from build123d import *

# Parameters (mm, degrees)
BOSS_EXTRUDE1_DEPTH                                = 4
CUT_EXTRUDE1_DEPTH                                 = 3
CUT_EXTRUDE2_DEPTH                                 = 58.329679868
F_3_2_3_2_DIAMETER_HOLE1_D                         = 3.2
F_3_2_3_2_DIAMETER_HOLE1_DEPTH                     = 6
CBORE_FOR_M3_5_HEX_HEAD_MACHINE_SCREW1_D           = 4
CBORE_FOR_M3_5_HEX_HEAD_MACHINE_SCREW1_CBORE_D     = 8
CBORE_FOR_M3_5_HEX_HEAD_MACHINE_SCREW1_CBORE_DEPTH = 4.5
CHAMFER1_SIZE                                      = 1.55
CHAMFER2_SIZE                                      = 0.799999982
CHAMFER2_SIZE2                                     = 0.800000027
CHAMFER3_SIZE                                      = 0.799999997
CHAMFER3_SIZE2                                     = 0.800000017
FILLET1_R                                          = 3
FILLET2_R                                          = 4.1
FILLET3_R                                          = 5
FILLET4_R                                          = 5.100000015


with BuildPart() as part:
    # Sketch1 → Boss-Extrude1 (new body)
    with BuildSketch(Plane(origin=(0, 4, 0), x_dir=(1, 0, 0), z_dir=(0, 1, 0))):
        with BuildLine():
            Line((19.999999925, -16.999999746), (19.999999925, 25.309401343))
            Line((19.999999925, 25.309401343), (29.980761952, 31.071796677))
            ThreePointArc((29.980761952, 31.071796677), (32.90896539, 41.999999919), (21.980762114, 44.92820323))
            Line((21.980762114, 44.92820323), (12.345871038, 39.365496274))
            ThreePointArc((12.345871038, 39.365496274), (0, 43.5), (-12.345871038, 39.365496274))
            Line((-12.345871038, 39.365496274), (-21.980762114, 44.92820323))
            ThreePointArc((-21.980762114, 44.92820323), (-32.908965409, 41.999999887), (-29.980761888, 31.071796639))
            Line((-29.980761888, 31.071796639), (-19.999999289, 25.3094011))
            Line((-19.999999289, 25.3094011), (-19.999999289, -16.999999746))
            Line((-19.999999289, -16.999999746), (19.999999925, -16.999999746))
        make_face()
    extrude(amount=-BOSS_EXTRUDE1_DEPTH)

    # Sketch2 → Cut-Extrude1 (cut)
    with BuildSketch(Plane(origin=(0, 4, 0), x_dir=(-1, 0, 0), z_dir=(0, 1, 0))):
        with BuildLine():
            Line((-4.968651732, -32.250000015), (4.968651732, -32.250000015))
            ThreePointArc((4.968651732, -32.250000015), (10.500000015, -23), (4.968651732, -13.749999985))
            Line((4.968651732, -13.749999985), (-4.968651732, -13.749999985))
            ThreePointArc((-4.968651732, -13.749999985), (-10.500000015, -23), (-4.968651732, -32.250000015))
        make_face()
    extrude(amount=-CUT_EXTRUDE1_DEPTH, mode=Mode.SUBTRACT)

    # Sketch3 → Cut-Extrude2 (cut, through all)
    with BuildSketch(Plane.XZ):
        with BuildLine():
            Line((4.71036092, -14.75), (-4.71036092, -14.75))
            ThreePointArc((-4.71036092, -14.75), (-9.5, -23), (-4.71036092, -31.25))
            Line((-4.71036092, -31.25), (4.71036092, -31.25))
            ThreePointArc((4.71036092, -31.25), (9.5, -23), (4.71036092, -14.75))
        make_face()
    extrude(amount=-CUT_EXTRUDE2_DEPTH, mode=Mode.SUBTRACT)

    # Sketch4 → Revolve1 (revolve)
    with BuildSketch(Plane(origin=(0, 0, -38), x_dir=(-1, 0, 0), z_dir=(0, 0, -1)), mode=Mode.PRIVATE) as revolve1_sk:
        Polygon((18.980762114, 4), (25.980762114, 4), (25.980762114, 6), (19.980762114, 6), (18.980762114, 5), align=None)
    revolve(revolve1_sk.sketch.rotate(Axis((-25.980762114, 4, -38), (0, 1, 0)), 270), axis=Axis((-25.980762114, 4, -38), (0, 1, 0)))

    # Sketch5 → Revolve2 (revolve)
    with BuildSketch(Plane(origin=(0, 0, 7), x_dir=(-1, 0, 0), z_dir=(0, 0, -1)), mode=Mode.PRIVATE) as revolve2_sk:
        Polygon((-7, 4), (0, 4), (0, 6), (-6, 6), (-7, 5), align=None)
    revolve(revolve2_sk.sketch.rotate(Axis((0, 4, 7), (0, 1, 0)), 180), axis=Axis((0, 4, 7), (0, 1, 0)))

    # Sketch6 → Revolve3 (revolve)
    with BuildSketch(Plane(origin=(0, 0, -38), x_dir=(-1, 0, 0), z_dir=(0, 0, -1)), mode=Mode.PRIVATE) as revolve3_sk:
        Polygon((-32.980762114, 4), (-25.980762114, 4), (-25.980762114, 6), (-31.980762114, 6), (-32.980762114, 5), align=None)
    revolve(revolve3_sk.sketch.rotate(Axis((25.980762114, 4, -38), (0, 1, 0)), 270), axis=Axis((25.980762114, 4, -38), (0, 1, 0)))

    # Ø3.2 (3.2) Diameter Hole1
    with Locations(Plane(origin=(0, 0, 0), x_dir=(-1, 0, 0), z_dir=(0, -1, 0))):
        with Locations((15.000000337, 33.000000191), (-14.999999663, 10.500000191), (15.000000337, -11.999999809), (-14.999999663, -11.999999809), (15.000000337, 10.500000191), (-14.999999663, 33.000000191)):
            Hole(F_3_2_3_2_DIAMETER_HOLE1_D / 2, depth=F_3_2_3_2_DIAMETER_HOLE1_DEPTH)

    # CBORE for M3.5 Hex Head Machine Screw1 (through all)
    with Locations(Plane(origin=(0, 0, 0), x_dir=(-1, 0, 0), z_dir=(0, -1, 0))):
        with Locations((0, -7), (-25.980762114, 38), (25.980762114, 38)):
            CounterBoreHole(CBORE_FOR_M3_5_HEX_HEAD_MACHINE_SCREW1_D / 2, CBORE_FOR_M3_5_HEX_HEAD_MACHINE_SCREW1_CBORE_D / 2, CBORE_FOR_M3_5_HEX_HEAD_MACHINE_SCREW1_CBORE_DEPTH)

    # Chamfer1
    chamfer1_edges = [part.edges().sort_by_distance(p)[0] for p in [
        (13.399999663, 0, -10.500000191),
        (-16.600000337, 0, -33.000000191),
        (13.399999663, 0, -33.000000191),
        (-16.600000337, 0, -10.500000191),
        (13.399999663, 0, 11.999999809),
        (-16.600000337, 0, 11.999999809),
    ]]
    chamfer(chamfer1_edges, length=CHAMFER1_SIZE)

    # Chamfer2
    chamfer2_edges = [part.edges().sort_by_distance(p)[0] for p in [
        (-19.999999289, 2, 16.999999746),
    ]]
    chamfer2_side = [part.faces().sort_by_distance(p)[0] for p in [
        (3.18e-07, 2, 16.999999746),
    ]]
    chamfer(chamfer2_edges, length=CHAMFER2_SIZE, length2=CHAMFER2_SIZE2, reference=chamfer2_side[0])

    # Chamfer3
    chamfer3_edges = [part.edges().sort_by_distance(p)[0] for p in [
        (19.999999925, 2, 16.999999746),
    ]]
    chamfer3_side = [part.faces().sort_by_distance(p)[0] for p in [
        (0.400000309, 2, 16.999999746),
    ]]
    chamfer(chamfer3_edges, length=CHAMFER3_SIZE, length2=CHAMFER3_SIZE2, reference=chamfer3_side[0])

    # Fillet1
    fillet1_edges = [part.edges().sort_by_distance(p)[0] for p in [
        (-12.345871038, 2, -39.365496274),
        (12.345871038, 2, -39.365496274),
    ]]
    fillet(fillet1_edges, radius=FILLET1_R)

    # Fillet2
    fillet2_edges = [part.edges().sort_by_distance(p)[0] for p in [
        (4.71036092, 0.5, -14.75),
        (4.71036092, 0.5, -31.25),
        (-4.71036092, 0.5, -31.25),
        (-4.71036092, 0.5, -14.75),
    ]]
    fillet(fillet2_edges, radius=FILLET2_R)

    # Fillet3
    fillet3_edges = [part.edges().sort_by_distance(p)[0] for p in [
        (-19.999999289, 2, -25.3094011),
        (19.999999925, 2, -25.309401343),
    ]]
    fillet(fillet3_edges, radius=FILLET3_R)

    # Fillet4
    fillet4_edges = [part.edges().sort_by_distance(p)[0] for p in [
        (4.968651732, 2.5, -32.250000015),
        (4.968651732, 2.5, -13.749999985),
        (-4.968651732, 2.5, -13.749999985),
        (-4.968651732, 2.5, -32.250000015),
    ]]
    fillet(fillet4_edges, radius=FILLET4_R)


solid = part.part
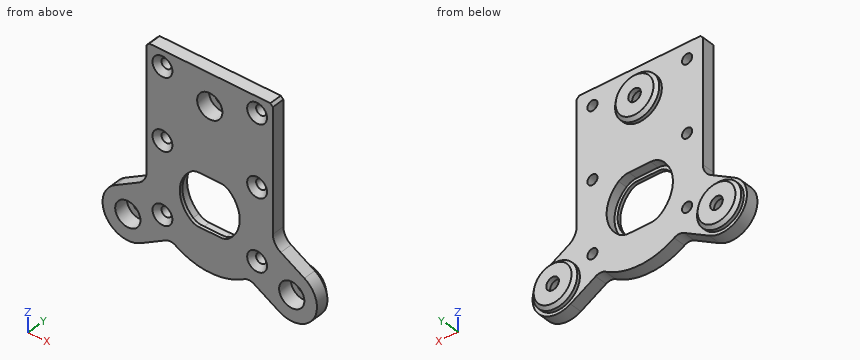
Geometry check sheet. Reference: the model listing, model coordinates, mm. Round coordinates to 2 decimals unless told otherwise and drop trailing zeros. Order: outer loops, then holes, each group sorted by start corner. A loop starts at its lowest first (then second) coordinate and runs counter-clockwise, first axis right, second up. Notation, with made-up numbers: M 49.25,-1.75 L 77.25,-1.75 A21 cw 77.25,34.25 Z; hole C 77,12 d6. An arc over 180 degrees is marked long. Answer in a Markdown table with one row per item. Add a question column.
Item 1: Depth check by flat-ended pin: pin 1 Ø19 at (x, z) = (11, -20.5) entering from +Y; pin 2 Ø3 at (x, z) = (-15, 12) entering from +Y; pin 3 Ø6.5 at (x, z) = (1.5, 6.5) entering from -Y; pin 4 Ø2.5 at (x, y) = (-1, 2.5) entering from -Z. Enter the tip coordinate at first touch or a pass-through.
Item 2: Material ranges on L1, parallel to X at y = 3.55, z = 12; L2, parallel to Z at x = -2.5, y = 2.4; L3, parallel to Y at x = -26.5, z = -40.5, recorded low to high. Write a range as [from, to].
Item 3: Sectioned sample at B-B, the plane z = 7. Enter the section's corners in (x, y).
Item 4: Sectioned sample at A-A, the plane x = 0. Enter the section's corners in (y, z), plus the area to 3 significant figures.
Item 5: Sectioned sample at C-C, the plane y = 2.55. State how many separate pieces and enclosed holes the cut face has, plus the area to 3 significant figures.
Filled in:
| question | item | result |
|---|---|---|
| 1 | pin 1 | stops at y = 4 |
| 1 | pin 2 | passes through |
| 1 | pin 3 | stops at y = 0 |
| 1 | pin 4 | stops at z = -43.5 |
| 2 | L1 | x = [-20, -16.6], [-13.4, 13.4], [16.6, 20] |
| 2 | L2 | z = [-43.35, -32.25], [-13.75, 3.88], [10.12, 17] |
| 2 | L3 | y = [4.5, 6] |
| 3 | outline | M -20,0 L -4,0 L -4,4.5 L -2,4.5 L -2,6 L -6,6 L -7,5 L -7,4 L -20,4 Z; M 2,4.5 L 4,4.5 L 4,0 L 20,0 L 20,4 L 7,4 L 7,5 L 6,6 L 2,6 Z |
| 4 | outline | M 0,-43.5 L 4,-43.5 L 4,-32.25 L 1,-32.25 L 1,-31.25 L 0,-31.25 Z; M 0,-14.75 L 1,-14.75 L 1,-13.75 L 4,-13.75 L 4,0 L 5,0 L 6,1 L 6,5 L 4.5,5 L 4.5,3 L 0,3 Z; M 0,11 L 4.5,11 L 4.5,9 L 6,9 L 6,13 L 5,14 L 4,14 L 4,17 L 0,17 Z |
| 4 | area | 155 mm² |
| 5 | separate pieces | 1 |
| 5 | enclosed holes | 10 |
| 5 | area | 2,260 mm² |
